Can you work these out from the model? Positions are in its coordinate system, mm. Face numbers are marked on the shaded views. A direction names the side the tool comes from. Coordinates: 2 decimals unless noted, no trailing zeros. Order: outer loops, then holes, each group sorted by start corner. A loop starts at its lowest first (then second) coordinate and runs counter-clockwise, first axis right, second up. Notation, with made-up numbers: M 8,-28.75 L 25,-28.75 A21 cw 25,6.25 Z; hole C 28.25,82.5 d2. An arc over 180 degrees is marked long. Answer as a JSON object with one key per item and string values.
Autodesk Inventor part; units mm, degrees
ref_plane "YZ Plane" through (0, 0, 0) normal (1, 0, 0) x (0, 1, 0)
ref_plane "XZ Plane" through (0, 0, 0) normal (0, 1, 0) x (-1, 0, 0)
ref_plane "XY Plane" through (0, 0, 0) normal (0, 0, 1) x (1, 0, 0)
sketch "Sketch1" plane through (0, 0, 0) normal (0, 0, 1) x (1, 0, 0)
  circle A0 centre (0, 0) radius 30
  dimension "d0" = 60
extrude "Extrusion1" add sketch "Sketch1" along normal blind 50
sketch "Sketch2" plane through (0, 0, 50) normal (0, 0, 1) x (1, 0, 0)
  circle A0 centre (0, 0) radius 30 construction
  line L0 (30, 0) -> (28.75, 0) construction
  line L1 (28.75, 16.5201) -> (34.9612, 16.5201)
  line L2 (34.9612, 16.5201) -> (34.9612, -18.249)
  line L3 (34.9612, -18.249) -> (28.75, -18.249)
  line L4 (28.75, -18.249) -> (28.75, 16.5201)
  dimension "d3" = 1.25
extrude "Extrusion2" cut sketch "Sketch2" against normal through all
sketch "Sketch3" plane through (28.75, -8.5696, 50) normal (1, 0, 0) x (0, 0, -1)
  line L0 (0, 38.5696) -> (0, -21.4304) construction
  line L1 (0, 8.5696) -> (14, 8.5696) construction
  circle A0 centre (14, 8.5696) radius 8.5
  point P0 (50, 8.5696)
  dimension "d6" = 14
  dimension "d7" = 17
extrude "Extrusion3" add sketch "Sketch3" along normal blind 3
sketch "Sketch4" plane through (28.75, -8.5696, 50) normal (1, 0, 0) x (0, 0, -1)
  line L0 (0, 0) -> (0, 17.1391)
  line L1 (0, 8.5696) -> (35, 8.5696) construction
  circle A0 centre (35, 8.5696) radius 8.5
  point P0 (50, 8.5696)
  dimension "d10" = 35
  dimension "d11" = 17
extrude "Extrusion4" add sketch "Sketch4" along normal blind 3
sketch "Sketch5" plane through (31.75, 0, 36) normal (1, 0, 0) x (0, 0, -1)
  circle A0 centre (0, 0) radius 8.5
  circle A1 centre (0, 0) radius 4.35
  circle A2 centre (21, 0) radius 8.5
  line L0 (12.5, 0) -> (21, 0)
  circle A3 centre (21, 0) radius 4.35
  point P0 (36, 0)
  dimension "d14" = 8.7
  dimension "d15" = 8.7
extrude "Extrusion5" add sketch "Sketch5" along normal blind 16 contours A1 | A3
sketch "Sketch6" plane through (28.75, -8.5696, 50) normal (1, 0, 0) x (0, 0, -1)
  line L0 (25, 8.5696) -> (29.25, 8.5696) construction
  line L1 (29.25, 8.5696) -> (29.25, 5.3196) construction
  line L2 (29.25, 5.3196) -> (20.75, 5.3196)
  line L3 (20.75, 5.3196) -> (20.75, 11.8196)
  line L4 (20.75, 11.8196) -> (29.25, 11.8196)
  line L5 (29.25, 11.8196) -> (29.25, 5.3196)
  point P0 (50, 8.5696)
  dimension "d18" = 4.25
  dimension "d19" = 3.25
  dimension "d20" = 8.5
  dimension "d21" = 6.5
extrude "Extrusion6" cut sketch "Sketch6" against normal through all
sketch "Sketch7" plane through (28.75, -8.5696, 50) normal (1, 0, 0) x (0, 0, -1)
  line L0 (29.25, 5.3196) -> (27.1459, 5.3196)
  line L1 (29.25, 5.3196) -> (20.75, 5.3196)
  line L2 (20.75, 5.3196) -> (20.75, 11.8196)
  line L3 (20.75, 11.8196) -> (29.25, 11.8196)
  line L4 (29.25, 11.8196) -> (29.25, 5.3196)
  point P0 (50, 8.5696)
  dimension "d24" = 8.5
  dimension "d25" = 6.5
extrude "Extrusion7" add sketch "Sketch7" against normal blind 55
properties part number "reservoir pump combo pump"
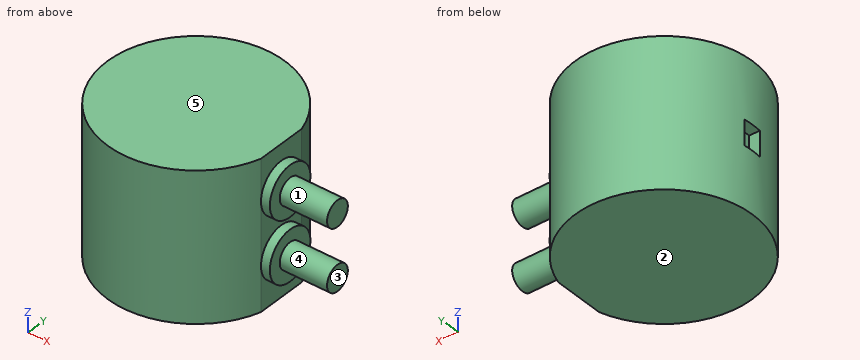
Item 1: Which directions (+Z, -Z, +X, -X, +Y, -Y) give clear straight access to the entire face, cutting with the end or side of a thin tool? Please do the marked faces 1 and 2.
Answers follow:
{"face 1": "+X", "face 2": "-Z, +X, -X, +Y, -Y"}
Item 2: I want a section at B-B, the plane z = 36. Write out the boundary of the cut face in (x, y).
Answers follow:
{"outline": "M 28.75,-8.57 L 28.75,-8.5 L 31.75,-8.5 L 31.75,-4.35 L 47.75,-4.35 L 47.75,4.35 L 31.75,4.35 L 31.75,8.5 L 28.75,8.5 L 28.75,8.57 A30 ccw long Z"}
Item 3: If we mould it in two halves opening along Z, with no side actions, what happens to the marked faces 3, 4 and 5? For each: pulls with the +Z half, pulls with the -Z half, needs draft (parallel to the pull), parting line crosses it, or undercut.
Answers follow:
{"face 3": "needs draft", "face 4": "undercut", "face 5": "pulls with the +Z half"}
Item 4: I want a section at D-D, the plane z = 14. Write out the boundary of the cut face in (x, y), plus the area to 3 significant figures.
Answers follow:
{"outline": "M 28.75,-8.57 L 28.75,-8.44 L 31.75,-8.44 L 31.75,-4.23 L 47.75,-4.23 L 47.75,4.23 L 31.75,4.23 L 31.75,8.44 L 28.75,8.44 L 28.75,8.57 A30 ccw long Z", "area": "3,000 mm^2"}
Item 5: I want a section at C-C, the plane x = -21. Write out the boundary of the cut face in (y, z), plus the area to 3 significant figures.
Answers follow:
{"outline": "M -21.42,0 L 21.42,0 L 21.42,50 L -21.42,50 Z", "area": "2,140 mm^2"}
Item 6: Please list where these lines run through material, in increasing order: line 1 (Y direction, x = -1, z = 25); line 2 (Y direction, x = -10.5, z = 41); line 3 (X direction, y = 13, z = 20).
Answers follow:
{"line 1": "y = -29.98 to 29.98", "line 2": "y = -28.1 to 28.1", "line 3": "x = -27.04 to 27.04"}
Item 7: I'm going to push flat-ended pins straight in: pin 1 (10 mm diameter, centred on y = 8, z = 44.5, fed in from +X); pin 2 (1 mm diameter, centred on x = -18.5, z = 42, fed in from +Y); pin 3 (7 mm diameter, centred on y = -0.5, z = 23.5, fed in from -X); pin 4 (2 mm diameter, centred on x = -15.5, z = 19.5, fed in from +Y). Where does each tip first touch, or does it pass through?
Answers follow:
{"pin 1": "stops at x = 31.75", "pin 2": "stops at y = 24", "pin 3": "stops at x = -30", "pin 4": "stops at y = 26.26"}
Item 8: I want a section at A-A, the plane y = 0. Write out the boundary of the cut face in (x, z), plus the area to 3 significant figures.
Answers follow:
{"outline": "M -30,0 L 28.75,0 L 28.75,6.5 L 31.75,6.5 L 31.75,10.65 L 47.75,10.65 L 47.75,19.35 L 31.75,19.35 L 31.75,23.5 L 28.75,23.5 L 28.75,27.5 L 31.75,27.5 L 31.75,31.65 L 47.75,31.65 L 47.75,40.35 L 31.75,40.35 L 31.75,44.5 L 28.75,44.5 L 28.75,50 L -30,50 L -30,29.25 L -26.25,29.25 L -26.25,20.75 L -30,20.75 Z", "area": "3,290 mm^2"}
